Read the model definition and answer for the solid it produces. Units are mm, in the model's axes. Face numbers are marked on the shaded views. A direction names the side the tool comes from. Give positions to 0.01 mm unless a question says otherwise; leave off trailing zeros. Order: outer loops, then holes, each group sorted by start corner. A loop starts at its lowest first (then second) coordinate and runs counter-clockwise, first axis right, second up. Notation, with made-up numbers: M 45.5,-36 L 102.5,-36 A19 ccw 102.5,-32 Z; hole C 81,85.5 d8. An arc over 180 degrees is marked long. One line per item, written item: value. Start each with the question number.
from build123d import *

# Parameters (mm, degrees)
CYLINDER298_R     = 1
CYLINDER298_DEPTH = 20
CYLINDER299_R     = 1
CYLINDER299_DEPTH = 20
BOX220_W          = 28
BOX220_H          = 1
BOX220_DEPTH      = 8
BOX197_W          = 21
BOX197_H          = 19
BOX197_DEPTH      = 8
BOX221_W          = 18
BOX221_H          = 27
BOX221_DEPTH      = 5.5
CYLINDER296_R     = 1.6
CYLINDER296_DEPTH = 10
CYLINDER297_R     = 1.6
CYLINDER297_DEPTH = 10
BOX224_W          = 69.8
BOX224_H          = 38.8
BOX224_DEPTH      = 4
CYLINDER300_R     = 2.6
CYLINDER300_DEPTH = 10
CYLINDER301_R     = 2.6
CYLINDER301_DEPTH = 10
BOX226_W          = 11
BOX226_H          = 17
BOX226_DEPTH      = 6
BOX227_W          = 4
BOX227_H          = 8
BOX227_DEPTH      = 11
BOX232_W          = 10
BOX232_H          = 10
BOX232_DEPTH      = 10
BOX222_W          = 10
BOX222_H          = 44
BOX222_DEPTH      = 3
CYLINDER295_R     = 8
CYLINDER295_DEPTH = 7
CYLINDER294_R     = 8
CYLINDER294_DEPTH = 7
BOX225_W          = 31
BOX225_H          = 15
BOX225_DEPTH      = 9
FILLET121_R       = 3
BOX223_W          = 13
BOX223_H          = 27
BOX223_DEPTH      = 2.5


with BuildPart() as zylinder300:
    # Cylinder298 → Cylinder298 (new body)
    with BuildSketch(Plane(origin=(22.5, 23, 30.5), x_dir=(1, 0, 0), z_dir=(0, -1, 0))):
        Circle(CYLINDER298_R)
    extrude(amount=CYLINDER298_DEPTH)


with BuildPart() as zylinder301:
    # Cylinder299 → Cylinder299 (new body)
    with BuildSketch(Plane(origin=(-1.5, 23, 30.5), x_dir=(1, 0, 0), z_dir=(0, -1, 0))):
        Circle(CYLINDER299_R)
    extrude(amount=CYLINDER299_DEPTH)


with BuildPart() as obj1:
    # Box220 → Box220 (new body)
    with BuildSketch(Plane(origin=(-3, 5, 26.5), x_dir=(1, 0, 0), z_dir=(0, 0, 1))):
        with Locations((14, 0.5)):
            Rectangle(BOX220_W, BOX220_H)
    extrude(amount=BOX220_DEPTH)


with BuildPart() as fusion207:
    # Box197 → Box197 (new body)
    with BuildSketch(Plane.XY.offset(26.5)):
        with Locations((10.5, 9.5)):
            Rectangle(BOX197_W, BOX197_H)
    extrude(amount=BOX197_DEPTH)

    # Fusion206: union obj1
    add(obj1.part)

    # Fusion207: union Zylinder300, Zylinder301
    add(zylinder300.part)
    add(zylinder301.part)


with BuildPart() as fusion207_1:
    # Fusion207 placement: moved
    add(fusion207.part.moved(Location((19.5, 1, -3.75))))


with BuildPart() as obj2:
    # Box221 → Box221 (new body)
    with BuildSketch(Plane(origin=(14.5, -13.5, 15), x_dir=(1, 0, 0), z_dir=(0, 0, 1))):
        with Locations((9, 13.5)):
            Rectangle(BOX221_W, BOX221_H)
    extrude(amount=BOX221_DEPTH)


with BuildPart() as zylinder298:
    # Cylinder296 → Cylinder296 (new body)
    with BuildSketch(Plane(origin=(25.5, -17.5, 12.25), x_dir=(1, 0, 0), z_dir=(0, 0, 1))):
        Circle(CYLINDER296_R)
    extrude(amount=CYLINDER296_DEPTH)


with BuildPart() as zylinder299:
    # Cylinder297 → Cylinder297 (new body)
    with BuildSketch(Plane(origin=(25.5, 17.5, 13), x_dir=(1, 0, 0), z_dir=(0, 0, 1))):
        Circle(CYLINDER297_R)
    extrude(amount=CYLINDER297_DEPTH)


with BuildPart() as board005:
    # Box224 → Box224 (new body)
    with BuildSketch(Plane(origin=(-42.5, -19.4, 16), x_dir=(1, 0, 0), z_dir=(0, 0, 1))):
        with Locations((34.9, 19.4)):
            Rectangle(BOX224_W, BOX224_H)
    extrude(amount=BOX224_DEPTH)


with BuildPart() as zylinder302:
    # Cylinder300 → Cylinder300 (new body)
    with BuildSketch(Plane(origin=(25.5, -17.5, 21.5), x_dir=(1, 0, 0), z_dir=(0, 0, 1))):
        Circle(CYLINDER300_R)
    extrude(amount=CYLINDER300_DEPTH)


with BuildPart() as zylinder303:
    # Cylinder301 → Cylinder301 (new body)
    with BuildSketch(Plane(origin=(25.5, 17.5, 21.5), x_dir=(1, 0, 0), z_dir=(0, 0, 1))):
        Circle(CYLINDER301_R)
    extrude(amount=CYLINDER301_DEPTH)


with BuildPart() as obj3:
    # Box226 → Box226 (new body)
    with BuildSketch(Plane(origin=(10.5, -22.5, 17.5), x_dir=(1, 0, 0), z_dir=(0, 0, 1))):
        with Locations((5.5, 8.5)):
            Rectangle(BOX226_W, BOX226_H)
    extrude(amount=BOX226_DEPTH)


with BuildPart() as obj4:
    # Box227 → Box227 (new body)
    with BuildSketch(Plane(origin=(36.5, 18.25, 23.5), x_dir=(1, 0, 0), z_dir=(0, 0, 1))):
        with Locations((2, 4)):
            Rectangle(BOX227_W, BOX227_H)
    extrude(amount=BOX227_DEPTH)


with BuildPart() as obj5:
    # Box232 → Box232 (new body)
    with BuildSketch(Plane(origin=(28.75, -6.75, 16.25), x_dir=(1, 0, 0), z_dir=(0, 0, 1))):
        with Locations((5, 5)):
            Rectangle(BOX232_W, BOX232_H)
    extrude(amount=BOX232_DEPTH)


with BuildPart() as fusion204:
    # Box222 → Box222 (new body)
    with BuildSketch(Plane(origin=(8.75, -22.5, 17.5), x_dir=(1, 0, 0), z_dir=(0, 0, 1))):
        with Locations((5, 22)):
            Rectangle(BOX222_W, BOX222_H)
    extrude(amount=BOX222_DEPTH)

    # Fusion204: union obj2, Zylinder298, Zylinder299, board005, Zylinder302, Zylinder303, obj3, obj4, obj5
    add(obj2.part)
    add(zylinder298.part)
    add(zylinder299.part)
    add(board005.part)
    add(zylinder302.part)
    add(zylinder303.part)
    add(obj3.part)
    add(obj4.part)
    add(obj5.part)


with BuildPart() as zylinder297:
    # Cylinder295 → Cylinder295 (new body)
    with BuildSketch(Plane(origin=(23.75, -13, 16), x_dir=(1, 0, 0), z_dir=(0, 0, 1))):
        Circle(CYLINDER295_R)
    extrude(amount=CYLINDER295_DEPTH)


with BuildPart() as zylinder296:
    # Cylinder294 → Cylinder294 (new body)
    with BuildSketch(Plane(origin=(23.75, 13, 16), x_dir=(1, 0, 0), z_dir=(0, 0, 1))):
        Circle(CYLINDER294_R)
    extrude(amount=CYLINDER294_DEPTH)


with BuildPart() as fillet121:
    # Box225 → Box225 (new body)
    with BuildSketch(Plane(origin=(14.5, 7, 20.75), x_dir=(1, 0, 0), z_dir=(0, 0, 1))):
        with Locations((15.5, 7.5)):
            Rectangle(BOX225_W, BOX225_H)
    extrude(amount=BOX225_DEPTH)

    # Fillet121
    fillet121_edges = [fillet121.edges().sort_by_distance(p)[0] for p in [
        (14.5, 22, 25.25),
        (45.5, 22, 25.25),
    ]]
    fillet(fillet121_edges, radius=FILLET121_R)


with BuildPart() as cut141:
    # Box223 → Box223 (new body)
    with BuildSketch(Plane(origin=(18.75, -13.5, 20.5), x_dir=(1, 0, 0), z_dir=(0, 0, 1))):
        with Locations((6.5, 13.5)):
            Rectangle(BOX223_W, BOX223_H)
    extrude(amount=BOX223_DEPTH)

    # Fusion205: union Zylinder297, Zylinder296, Fillet121
    add(zylinder297.part)
    add(zylinder296.part)
    add(fillet121.part)

    # Cut140: cut Fusion204
    add(fusion204.part, mode=Mode.SUBTRACT)

    # Cut141: cut Fusion207
    add(fusion207_1.part, mode=Mode.SUBTRACT)


with BuildPart() as cut141_1:
    # Cut141 placement: moved
    add(cut141.part.moved(Location((0, 0, 2))))


solid = cut141_1.part
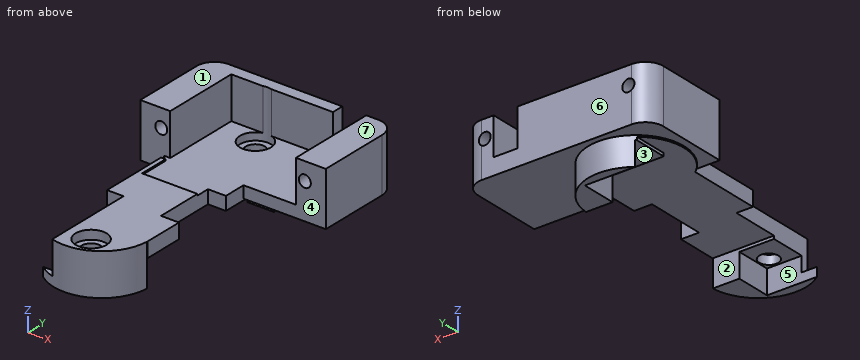
Q1. Determine the mould class of the marked faces 5, 6 and 7 for opening direction Y: released by +Y, released by -Y, zero draft, split by the parting line, or undercut.
Q2. Find section B-B, the plane y = 17.5. Give the vertices of the cut face in (x, z), then the cut area to 3 significant figures.
Q3. A tool of negligible diameter and unlimited length cuts with its end or side. For the marked faces 1, 2, 3 and 4, from which of +Z, -Z, +X, -X, +Y, -Y can it reach the whole face along a straight path? Write none if from no direction.
Q4. Consider probe 1 along Y at (x, z) = (25.5, 23); probe 2 along Y at (x, z) = (24, 20.75); probe 3 along Y at (x, z) = (25.5, 24.4). Determine where each line is inside the solid, lowest interval first.
Q5. Find section D-D, the plane y = 13. Give the vertices of the cut face in (x, z), then the cut area to 3 significant figures.
Q6. Find section A-A, the plane x = 42. Give the vertices of the cut face in (y, z).
Q7. Find section C-C, the plane z = 30.75. Give the vertices of the cut face in (x, y), then the cut area to 3 significant figures.
Q8. Each of these flat-tipped pins is pushed along its axis until it touches: pin 1 (8 mm diameter, centred on y = -7.5, z = 28.5, fed in from +X); pin 2 (3 mm diameter, centred on x = 20.5, z = 23.5, fed in from -Y); pin 3 (1 mm diameter, centred on x = 18.5, z = 24, fed in from -Y). Where does it stop, or does it pass through?
Evaluation:
1. face 5: undercut
1. face 6: released by +Y
1. face 7: zero draft
2. outline: M 14.5,22.75 L 17.14,22.75 L 17.14,22.5 L 18.75,22.5 L 18.75,22 L 23.9,22 L 23.9,23.5 L 22.9,23.5 L 22.9,24.75 L 19.5,24.75 L 19.5,31.75 L 14.5,31.75 Z; M 27.1,22 L 27.3,22 L 27.3,18 L 30.36,18 L 30.36,22.75 L 45.5,22.75 L 45.5,31.75 L 40.5,31.75 L 40.5,24.75 L 28.1,24.75 L 28.1,23.5 L 27.1,23.5 Z; hole C 18,28.75 d2; hole C 42,28.75 d2
2. area: 136 mm2
3. face 1: +Z, +X, -X, +Y, -Y
3. face 2: -Z, +X, -X
3. face 3: -Z, -X
3. face 4: +Z, -Z, +X, -Y
4. probe 1: -20.81 to -19.1, -15.9 to 15.9, 19.1 to 22
4. probe 2: -21 to -19.4, 19.4 to 21
4. probe 3: -20.81 to -20.1, -14.9 to 14.9, 20.1 to 22
5. outline: M 14.5,22.75 L 15.75,22.75 L 15.75,22.5 L 31.75,22.5 L 31.75,22.75 L 45.5,22.75 L 45.5,31.75 L 40.5,31.75 L 40.5,24.75 L 19.5,24.75 L 19.5,31.75 L 14.5,31.75 Z; hole C 18,28.75 d2; hole C 42,28.75 d2
5. area: 130 mm2
6. outline: M 7,22.75 L 22,22.75 L 22,27.75 L 7,27.75 Z; M 7,29.75 L 22,29.75 L 22,31.75 L 7,31.75 Z
7. outline: M 14.5,7 L 19.5,7 L 19.5,20 L 24.79,20 A2.6 cw 26.21,20 L 36.5,20 L 36.5,22 L 17.5,22 A3 ccw 14.5,19 Z; M 40.5,7 L 45.5,7 L 45.5,19 A3 ccw 42.5,22 L 40.5,22 Z
7. area: 180 mm2
8. pin 1: x = 31.75
8. pin 2: y = -20.81
8. pin 3: y = -5.5
